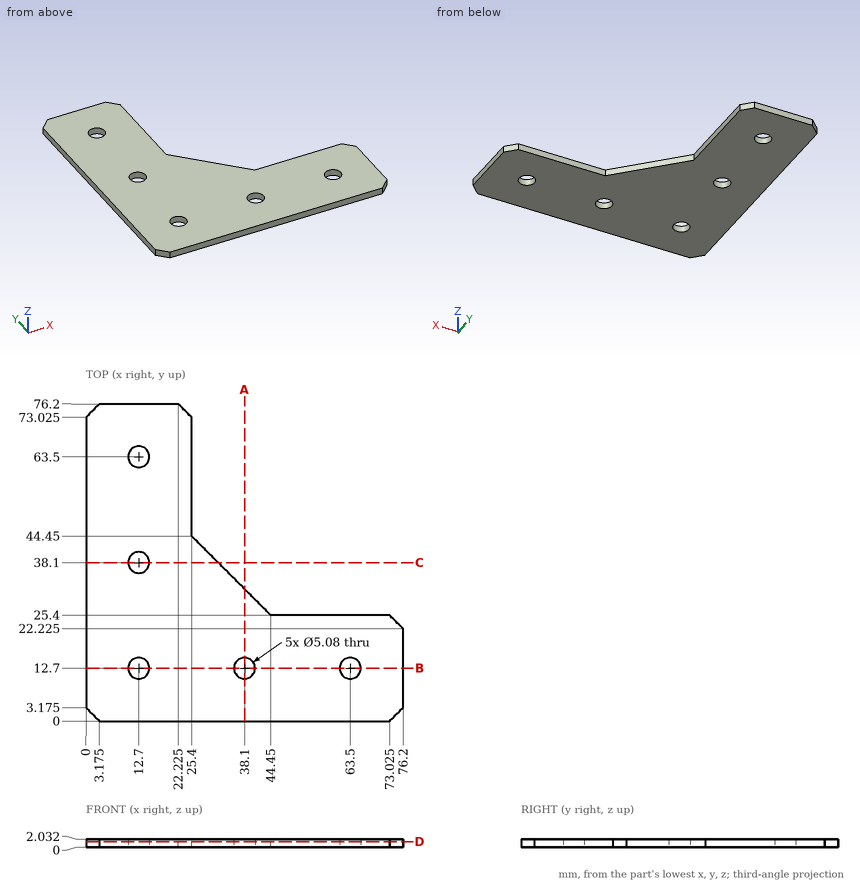
Geometry: see drawing. Coordinates: mm, zero at the bounding-box minimum. Give positions to 0.01 mm unless a question says otherwise; leave off trailing zeros. Order: outer loops, then holes, each group sorted by start corner. A loop starts at its lowest first (then second) coordinate and runs counter-clockwise, first axis right, second up. Notation, with made-up numbers: (-14.5, 12) - (1.5, 12) arc R19 cw to (1.5, 31) - close; hole circle Ø11 at (20.5, 3). An arc over 180 degrees is marked (long way). Write each question's results on one line, items separated by ' | '.
Item 1: Material intervals for line 1 along Y through (x, z) = (12.7, 1.2); line 2 along Y through (x, z) = (63.5, 0.8); line 3 along X through (y, z) = (10.5, 0.6), sorted ascending.
A:
line 1: y = 0 to 10.16, 15.24 to 35.56, 40.64 to 60.96, 66.04 to 76.2 | line 2: y = 0 to 10.16, 15.24 to 25.4 | line 3: x = 0 to 11.43, 13.97 to 36.83, 39.37 to 62.23, 64.77 to 76.2
Item 2: Section D-D (z = 1.4). Return loops of the section in (x, y) (3 decimals), and give its area (3 significant figures).
A:
outline: (0, 3.175) - (3.175, 0) - (73.025, 0) - (76.2, 3.175) - (76.2, 22.225) - (73.025, 25.4) - (44.45, 25.4) - (25.4, 44.45) - (25.4, 73.025) - (22.225, 76.2) - (3.175, 76.2) - (0, 73.025) - close; hole circle Ø5.08 at (12.7, 12.7); hole circle Ø5.08 at (12.7, 38.1); hole circle Ø5.08 at (12.7, 63.5); hole circle Ø5.08 at (38.1, 12.7); hole circle Ø5.08 at (63.5, 12.7) | area: 3,280 mm^2
Item 3: Section B-B (y = 12.7). Return loops of the section in (x, z), and give its area (3 significant figures).
A:
outline: (0, 0) - (10.16, 0) - (10.16, 2.03) - (0, 2.03) - close; (15.24, 0) - (35.56, 0) - (35.56, 2.03) - (15.24, 2.03) - close; (40.64, 0) - (60.96, 0) - (60.96, 2.03) - (40.64, 2.03) - close; (66.04, 0) - (76.2, 0) - (76.2, 2.03) - (66.04, 2.03) - close | area: 124 mm^2
Item 4: Contact query for a flat-ended pin moving along its axis: pin 1 Ø3 at (x, y) = (12.7, 12.7) entering from -Z. Output: stop coordinate, or through.
A:
pin 1: passes through
Item 5: Section A-A (x = 38.1). Return loops of the section in (y, z), and give its area (3 significant figures).
A:
outline: (0, 0) - (10.16, 0) - (10.16, 2.03) - (0, 2.03) - close; (15.24, 0) - (31.75, 0) - (31.75, 2.03) - (15.24, 2.03) - close | area: 54.2 mm^2
